Autodesk Inventor part; units mm, degrees
ref_plane "YZ Plane" through (0, 0, 0) normal (1, 0, 0) x (0, 1, 0)
ref_plane "XZ Plane" through (0, 0, 0) normal (0, 1, 0) x (-1, 0, 0)
ref_plane "XY Plane" through (0, 0, 0) normal (0, 0, 1) x (1, 0, 0)
sketch "Sketch1" plane through (0, 0, 0) normal (0, 0, 1) x (1, 0, 0)
  line L0 (60, 13.5) -> (60, 0) construction
  line L1 (60, 0) -> (60, 34)
  line L2 (60, 34) -> (78, 34)
  line L3 (78, 34) -> (78, 0)
  line L4 (78, 0) -> (78, 21)
  line L5 (78, 21) -> (99, 21)
  line L6 (99, 21) -> (99, 0)
  line L7 (99, 0) -> (99, 15)
  line L8 (99, 15) -> (110, 15)
  line L9 (110, 15) -> (110, 0)
  line L10 (110, 0) -> (110, 10)
  line L11 (110, 10) -> (130, 10)
  line L12 (130, 10) -> (130, 0)
  line L13 (130, 0) -> (130, 8)
  line L14 (130, 8) -> (144, 8)
  line L15 (144, 8) -> (144, 0)
  line L16 (144, 0) -> (144, 10)
  line L17 (144, 10) -> (176, 10)
  line L18 (176, 10) -> (176, 0)
  line L19 (0, 0) -> (225.6875, 0)
  dimension "d8" = 34
  dimension "d9" = 18
  dimension "d10" = 21
  dimension "d11" = 21
  dimension "d12" = 15
  dimension "d13" = 11
  dimension "d14" = 10
  dimension "d15" = 20
  dimension "d16" = 8
  dimension "d17" = 14
  dimension "d18" = 10
  dimension "d19" = 32
  dimension "d46" = 98
revolve "Revolution1" add sketch "Sketch1" angle 360 about axis through (0, 0, 0) along (1, 0, 0)
sketch "Sketch4" plane through (60, 0, 0) normal (-1, 0, 0) x (0, 0, 1)
  point P0 (0, 0)
properties part number "Sketch 2d terminado sin rotacion aun"
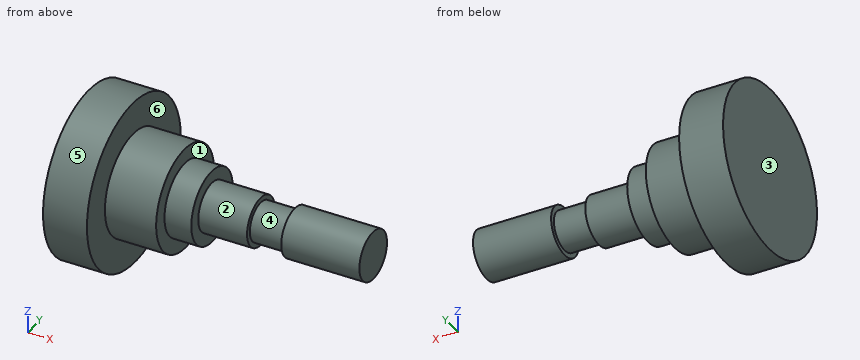
Build history of the part. All positions in model axes, mm. Face numbers are marked on the shaded views. A direction names the side the tool comes from. Give positions to 0.01 mm unless a question says otherwise; leave off trailing zeros. Loops run counter-clockwise (first coordinate to the right, second up) from the corner with the lowest first, then second, coordinate; pieces in that order, holes last.
Item 1: Flat gauge pins, fed straight in: pin 1 (5 mm diameter, centred on x = 132.5, y = 12.5, fed in from +Z); pin 2 (8 mm diameter, centred on x = 99, y = 3, fed in from -Z); pin 3 (6 mm diameter, centred on y = -9, z = 19.5, fed in from +X); pin 4 (4 mm diameter, centred on x = 143, y = 3, fed in from +Z). Where does each tip first touch, or does it go through?
Answers follow:
pin 1: passes through
pin 2: stops at z = -21
pin 3: stops at x = 99
pin 4: stops at z = 9.92
Item 2: Slice it at A-A, the plane y = 0. List the corners of the cut face in (x, z).
Answers follow:
outline: (60, -34) - (78, -34) - (78, -21) - (99, -21) - (99, -15) - (110, -15) - (110, -10) - (130, -10) - (130, -8) - (144, -8) - (144, -10) - (176, -10) - (176, 10) - (144, 10) - (144, 8) - (130, 8) - (130, 10) - (110, 10) - (110, 15) - (99, 15) - (99, 21) - (78, 21) - (78, 34) - (60, 34) - close
Item 3: Drill centre lines: line 1 (X direction, y = 13.5, z = 2.5); line 2 (X direction, y = 24.5, z = -20.5); line 3 (Z direction, x = 75, y = 23). Where is each one in solid material? Low to high.
Answers follow:
line 1: x = 60 to 110
line 2: x = 60 to 78
line 3: z = -25.04 to 25.04
Item 4: Slice it at B-B, the plane z = -12. List the corners of the cut face in (x, y).
Answers follow:
outline: (60, -31.81) - (78, -31.81) - (78, -17.23) - (99, -17.23) - (99, -9) - (110, -9) - (110, 9) - (99, 9) - (99, 17.23) - (78, 17.23) - (78, 31.81) - (60, 31.81) - close
Item 5: Slice it at C-C, the plane x = 153. List the corners of the cut face in (y, z).
Answers follow:
outline: circle Ø20 at (0, 0)
Item 6: Which spindle directions (+Z, -Z, +X, -X, +Y, -Y) get a long thin tool onto all of the face, cutting with end or side? Do the marked faces 5 and 6. Say none if no direction does.
Answers follow:
face 5: +X, -X
face 6: +X
Item 7: Pull direction X, two halves, no side cores. Call the marked faces 1, 2, 3 and 4: released by +X, released by -X, zero draft, split by the parting line, or undercut.
Answers follow:
face 1: released by +X
face 2: zero draft
face 3: released by -X
face 4: undercut
